Could you check a few things on this model? Use its own coordinates, in mm. A direction names the side the tool comes from. Coordinates: 2 decimals unless noted, no trailing zeros. Loops run counter-clockwise (first coordinate to the right, second up) from the corner with the lowest first, then second, coordinate; pieces in that order, holes last.
from build123d import *

# Parameters (mm, degrees)
SKETCH1_R           = 4.7625
SKETCH1_R_2         = 1.905
BOSS_EXTRUDE1_DEPTH = 4.7625


with BuildPart() as part:
    # Sketch1 → Boss-Extrude1 (new body)
    with BuildSketch(Plane(origin=(0, 0, 0), x_dir=(1, 0, 0), z_dir=(0, 1, 0))):
        with BuildLine():
            Line((10.16, 0), (40.64, 0))
            ThreePointArc((40.64, 0), (47.824204897, -2.975795103), (50.8, -10.16))
            Line((50.8, -10.16), (50.8, -16.51))
            Line((50.8, -16.51), (254, -16.51))
            Line((254, -16.51), (254, -67.31))
            Line((254, -67.31), (50.8, -67.31))
            Line((50.8, -67.31), (50.8, -73.66))
            ThreePointArc((50.8, -73.66), (47.824204897, -80.844204897), (40.64, -83.82))
            Line((40.64, -83.82), (10.16, -83.82))
            ThreePointArc((10.16, -83.82), (2.975795103, -80.844204897), (0, -73.66))
            Line((0, -73.66), (0, -50.8))
            Line((0, -50.8), (10.16, -50.8))
            ThreePointArc((10.16, -50.8), (19.05, -41.91), (10.16, -33.02))
            Line((10.16, -33.02), (0, -33.02))
            Line((0, -33.02), (0, -10.16))
            ThreePointArc((0, -10.16), (2.975795103, -2.975795103), (10.16, 0))
        make_face()
        with Locations(Location((10.16, -60.96, 0), (0, 0, 90))):
            Circle(SKETCH1_R, mode=Mode.SUBTRACT)
        with Locations(Location((10.16, -22.86, 0), (0, 0, 90))):
            Circle(SKETCH1_R, mode=Mode.SUBTRACT)
        with Locations(Location((35.56, -71.12, 0), (0, 0, 90))):
            Circle(SKETCH1_R_2, mode=Mode.SUBTRACT)
        with Locations(Location((35.56, -12.7, 0), (0, 0, 90))):
            Circle(SKETCH1_R_2, mode=Mode.SUBTRACT)
    boss_extrude1 = extrude(amount=BOSS_EXTRUDE1_DEPTH)

    # Mirror1: Boss-Extrude1 across plane
    add(boss_extrude1.mirror(Plane(origin=(254, 4.7625, 67.31), x_dir=(0, 0, 1), z_dir=(-1, 0, 0))))


solid = part.part
1) Imagine slicing it at C-C on x = 327.5. List the corners of the cut face in (y, z) for me, plus the area to 3 significant figures.
2) If I drill on L1, parallel to Z at x = 35.56, y = 3.6 (3 decimals); L2, parallel to Z at x = 472, y = 2; L3, parallel to X at y = 3.25, z = 22.86, over which ranges is the centre line in solid material (lowest first)?
3) Imagine slicing it at B-B on y = 3.5. State how many separate pieces and enclosed holes the cut face has, plus the area to 3 significant figures.
4) Imagine slicing it at A-A on z = 41.91. List the corners of the cut face in (x, y) for me, plus the area to 3 significant figures.
5) We'd pull the mould along Z, two halves only. Please class faces 4 (the cylindrical face through (488.952, 2.348, 42.105)), 5 (the cylindrical face through (47.903, 2.348, 80.765)), 6 (the cylindrical face through (19.048, 2.348, 42.105)), 7 (the cylindrical face through (2.897, 2.348, 3.055)): released by +Z, released by -Z, zero draft, split by the parting line, or undercut.
6) For faces 1 (the cylindrical face through (13.06, 2.35, 26.64)), 2 (the cylindrical face through (460.097, 2.348, 80.765)), 3 (the cylindrical face through (460.255, 2.348, 2.897)), which set-ups out of +Z, -Z, +X, -X, +Y, -Y let a thin tool reach every point of the face, with its end or its side?
7) Will these pins go through, and if not, where does the flat tip stop? pin 1 (2.5 mm diameter, centred on x = 472.44, z = 71.12, fed in from -Y); pin 2 (1.4 mm diameter, centred on x = 316, y = 2, fed in from +Z); pin 3 (1.4 mm diameter, centred on x = 501, y = 1.5, fed in from +Z); pin 4 (1.5 mm diameter, centred on x = 277.5, y = 3.5, fed in from -Z).
Solved:
1. outline: (0, 16.51) - (4.76, 16.51) - (4.76, 67.31) - (0, 67.31) - close
1. area: 242 mm2
2. L1: z = 0 to 10.795, 14.605 to 69.215, 73.025 to 83.82
2. L2: z = 0 to 10.85, 14.55 to 69.27, 72.97 to 83.82
2. L3: x = 0 to 5.4, 14.92 to 493.08, 502.6 to 508
3. separate pieces: 1
3. enclosed holes: 8
3. area: 28,000 mm2
4. outline: (19.05, 0) - (488.95, 0) - (488.95, 4.76) - (19.05, 4.76) - close
4. area: 2,240 mm2
5. face 4: undercut
5. face 5: released by +Z
5. face 6: undercut
5. face 7: released by -Z
6. face 1: +Y, -Y
6. face 2: +Z, +Y, -Y
6. face 3: -Z, +Y, -Y
7. pin 1: passes through
7. pin 2: stops at z = 67.31
7. pin 3: stops at z = 83.52
7. pin 4: stops at z = 16.51
